CAD build for the part. Positions are in the model's coordinates, mm. Face numbers are marked on the shaded views. A direction names the side the tool comes from. Coordinates: 2 decimals unless noted, no trailing zeros. Loops run counter-clockwise (first coordinate to the right, second up) from the corner with the lowest first, then second, coordinate; pieces in that order, holes last. Notation, with made-up numbers: (-34, 60) -> (-10, 60) arc R20 ccw to (-10, 77) -> close; hole circle Ø6 at (13.25, -3). An arc over 180 degrees is marked (long way). Write each question's results on one line, items separated by ' | '.
Autodesk Fusion 360 part; units mm, degrees
sketch "Sketch1" plane through (0, 0, 0) normal (0, 1, 0) x (1, 0, 0)
  circle A0 centre (0, 0) radius 1.75
  circle A1 centre (50, 0) radius 1.75
  circle A2 centre (0, -50) radius 1.75
  circle A3 centre (50, -50) radius 1.75
  circle A4 centre (25, -25) radius 4.5
  line L0 (-5, 5) -> (55, 5)
  line L1 (55, 5) -> (55, -55)
  line L2 (55, -55) -> (-5, -55)
  line L3 (-5, -55) -> (-5, 5)
  dimension "d1" = 50
  dimension "d2" = 50
  dimension "d3" = 3.5
  dimension "d4" = 3.5
  dimension "d5" = 3.5
  dimension "d6" = 3.5
  dimension "d7" = 9
extrude "Extrude1" add sketch "Sketch1" along normal blind 4 contours A4 | L0 L1 L2 L3
sketch "Sketch2" plane through (0, 4, 0) normal (0, 1, 0) x (-1, 0, 0)
  circle A0 centre (0, 0) radius 1.75
  circle A1 centre (-50, 0) radius 1.75
  circle A2 centre (0, 50) radius 1.75
  circle A3 centre (-50, 50) radius 1.75
  line L0 (5, 55) -> (-55, 55)
  line L1 (-55, 55) -> (-55, -5)
  line L2 (-55, -5) -> (5, -5)
  line L3 (5, -5) -> (5, 55)
  circle A4 centre (0, 0) radius 3.25
  circle A5 centre (-50, 0) radius 3.25
  circle A6 centre (0, 50) radius 3.25
  circle A7 centre (-50, 50) radius 3.25
  dimension "d10" = 6.5
  dimension "d11" = 6.5
  dimension "d12" = 6.5
  dimension "d13" = 6.5
extrude "Extrude2" add sketch "Sketch2" along normal blind 0.5 contours L0 L1 L2 L3
extrude "Extrude3" cut 1 faces at (-2.7314, 4, -0.2484) along direction (0, -1, 0) blind 2
extrude "Extrude4" cut 1 faces at (-2.7314, 4, 49.7516) along direction (0, -1, 0) blind 2
sketch "Sketch3" plane through (0, 4, 0) normal (0, 1, 0) x (-1, 0, 0)
  circle A0 centre (-50, 0) radius 3.25
  circle A1 centre (-50, 0) radius 1.75
extrude "Extrude5" cut sketch "Sketch3" against normal blind 2
extrude "Extrude6" cut 1 faces at (47.2686, 4, 49.7516) along direction (0, -1, 0) blind 2
sketch "Sketch4" plane through (0, 4.5, 0) normal (0, 1, 0) x (-1, 0, 0)
  circle A0 centre (-50, 50) radius 3.25
  circle A1 centre (-50, 0) radius 3.25
  circle A2 centre (0, 50) radius 3.25
  circle A3 centre (0, 0) radius 3.25
  line L0 (5, -5) -> (5, 55)
  line L1 (5, 55) -> (-55, 55)
  line L2 (-55, 55) -> (-55, -5)
  line L3 (-55, -5) -> (5, -5)
  line L4 (-24, 3) -> (-26, 3)
  line L5 (-10.0926, 8.7898) -> (-11.6247, 7.5042)
  line L6 (-3.1606, 22.1645) -> (-3.5079, 20.1949)
  line L7 (-6.4474, 36.866) -> (-5.4474, 35.134)
  line L8 (-18.4152, 46.0153) -> (-16.5359, 45.3312)
  line L9 (-33.4641, 45.3312) -> (-31.5848, 46.0153)
  line L10 (-44.5526, 35.134) -> (-43.5526, 36.866)
  line L11 (-46.4921, 20.1949) -> (-46.8394, 22.1645)
  line L12 (-38.3753, 7.5042) -> (-39.9074, 8.7898)
  circle A4 centre (-25, 25) radius 15
  line L13 (-11.6247, 7.5042) -> (-16.1457, 12.8921)
  line L14 (-14.6136, 14.1777) -> (-10.0926, 8.7898)
  line L15 (-24, 10.0334) -> (-24, 3)
  line L16 (-26, 3) -> (-26, 10.0334)
  line L17 (-33.8543, 12.8921) -> (-38.3753, 7.5042)
  line L18 (-39.9074, 8.7898) -> (-35.3864, 14.1777)
  line L19 (-39.5656, 21.4163) -> (-46.4921, 20.1949)
  line L20 (-46.8394, 22.1645) -> (-39.9129, 23.3859)
  line L21 (-38.4615, 31.6173) -> (-44.5526, 35.134)
  line L22 (-43.5526, 36.866) -> (-37.4615, 33.3493)
  line L23 (-31.0586, 38.722) -> (-33.4641, 45.3312)
  line L24 (-31.5848, 46.0153) -> (-29.1792, 39.4061)
  line L25 (-20.8208, 39.4061) -> (-18.4152, 46.0153)
  line L26 (-16.5359, 45.3312) -> (-18.9414, 38.722)
  line L27 (-12.5385, 33.3493) -> (-6.4474, 36.866)
  line L28 (-5.4474, 35.134) -> (-11.5385, 31.6173)
  line L29 (-10.0871, 23.3859) -> (-3.1606, 22.1645)
  line L30 (-3.5079, 20.1949) -> (-10.4344, 21.4163)
  line L31 (-25.8167, 5.0167) -> (-26, 3) construction
  arc A5 (-26, 5.025) -> (-25.8167, 5.0167) centre (-25, 25) ccw
  dimension "d27" = 30
extrude "Extrude7" add sketch "Sketch4" along normal blind 9.5 contours L4 A4 L15 L16 | A4 | L5 A4 L13 L14 | L12 A4 L17 L18 | L6 A4 L29 L30 | L11 A4 L19 L20 | L10 A4 L21 L22 | L7 A4 L27 L28 | L9 A4 L23 L24 | L8 A4 L25 L26
extrude "Extrude8" add 1 faces at (24.6667, 7.6667, 3) along direction (0, 0, -1) blind 2.5
chamfer "Chamfer1" distance 9.5 angle 45 1 edges at (25, 14, 0.5)
extrude "Extrude9" add 1 faces at (10.6033, 7.6667, 8.3613) along direction (-0.642788, 0, -0.766044) blind 2.5
extrude "Extrude10" add 1 faces at (3.2763, 7.6667, 21.508) along direction (-0.984808, 0, -0.173648) blind 2.5
extrude "Extrude11" add 1 faces at (6.1141, 7.6667, 36.2887) along direction (-0.866025, 0, 0.5) blind 2.5
extrude "Extrude12" add 1 faces at (17.7888, 7.6667, 45.7872) along direction (-0.34202, 0, 0.939693) blind 2.5
extrude "Extrude13" add 1 faces at (32.8377, 7.6667, 45.5592) along direction (0.34202, 0, 0.939693) blind 2.5
extrude "Extrude14" add 1 faces at (44.2192, 7.6667, 35.7113) along direction (0.866025, 0, 0.5) blind 2.5
extrude "Extrude15" add 1 faces at (46.6079, 7.6667, 20.8515) along direction (0.984808, 0, -0.173648) blind 2.5
extrude "Extrude16" add 1 faces at (38.886, 7.6667, 7.9328) along direction (0.642788, 0, -0.766044) blind 2.5
chamfer "Chamfer2" distance 9.5 angle 45 8 edges at (49.1278, 14, 20.7456) (40.7483, 14, 6.2319) (46.2176, 14, 37.25) (9.2517, 14, 6.2319) (33.3795, 14, 48.0225) (16.6205, 14, 48.0225) (3.7824, 14, 37.25) (0.8722, 14, 20.7456)
sketch "Sketch5" plane through (0, 14, 0) normal (0, 1, 0) x (-1, 0, 0)
  line L0 (-10.4015, 21.4105) -> (-10.0542, 23.3801)
  line L1 (-10.0542, 23.3801) -> (-10.0871, 23.3859)
  arc A0 (-10.0871, 23.3859) -> (-11.5385, 31.6173) centre (-25, 25) ccw
  line L2 (-11.5385, 31.6173) -> (-11.5096, 31.634)
  line L3 (-11.5096, 31.634) -> (-12.5096, 33.366)
  line L4 (-12.5096, 33.366) -> (-12.5385, 33.3493)
  arc A1 (-12.5385, 33.3493) -> (-18.9414, 38.722) centre (-25, 25) ccw
  line L5 (-18.9414, 38.722) -> (-18.93, 38.7534)
  line L6 (-18.93, 38.7534) -> (-20.8094, 39.4374)
  line L7 (-20.8094, 39.4374) -> (-20.8208, 39.4061)
  arc A2 (-20.8208, 39.4061) -> (-29.1792, 39.4061) centre (-25, 25) ccw
  line L8 (-29.1792, 39.4061) -> (-29.1906, 39.4374)
  line L9 (-29.1906, 39.4374) -> (-31.07, 38.7534)
  line L10 (-31.07, 38.7534) -> (-31.0586, 38.722)
  arc A3 (-31.0586, 38.722) -> (-37.4615, 33.3493) centre (-25, 25) ccw
  line L11 (-37.4615, 33.3493) -> (-37.4904, 33.366)
  line L12 (-37.4904, 33.366) -> (-38.4904, 31.634)
  line L13 (-38.4904, 31.634) -> (-38.4615, 31.6173)
  arc A4 (-38.4615, 31.6173) -> (-39.9129, 23.3859) centre (-25, 25) ccw
  line L14 (-39.9129, 23.3859) -> (-39.9458, 23.3801)
  line L15 (-39.9458, 23.3801) -> (-39.5985, 21.4105)
  line L16 (-39.5985, 21.4105) -> (-39.5656, 21.4163)
  arc A5 (-39.5656, 21.4163) -> (-35.3864, 14.1777) centre (-25, 25) ccw
  line L17 (-35.3864, 14.1777) -> (-35.4079, 14.1521)
  line L18 (-35.4079, 14.1521) -> (-33.8758, 12.8665)
  line L19 (-33.8758, 12.8665) -> (-33.8543, 12.8921)
  arc A6 (-33.8543, 12.8921) -> (-26, 10.0334) centre (-25, 25) ccw
  line L20 (-26, 10.0334) -> (-26, 10)
  line L21 (-26, 10) -> (-24, 10)
  line L22 (-24, 10) -> (-24, 10.0334)
  arc A7 (-24, 10.0334) -> (-16.1457, 12.8921) centre (-25, 25) ccw
  line L23 (-16.1457, 12.8921) -> (-16.1242, 12.8665)
  line L24 (-16.1242, 12.8665) -> (-14.5921, 14.1521)
  line L25 (-14.5921, 14.1521) -> (-14.6136, 14.1777)
  arc A8 (-14.6136, 14.1777) -> (-10.4344, 21.4163) centre (-25, 25) ccw
  line L26 (-10.4344, 21.4163) -> (-10.4015, 21.4105)
  circle A9 centre (-25, 25) radius 4.5
  dimension "d50" = 9
extrude "Extrude17" cut sketch "Sketch5" against normal blind 12 contours A9
chamfer "Chamfer3" distance 1 angle 45 1 edges at (29.1955, 14, 26.6273)
sketch "Sketch6" plane through (55, 0, 0) normal (1, 0, 0) x (0, 0, -1)
  line L0 (-55, 0) -> (5, 0)
  line L1 (5, 0) -> (5, 4.5)
  line L2 (5, 4.5) -> (-55, 4.5)
  line L3 (-55, 4.5) -> (-55, 0)
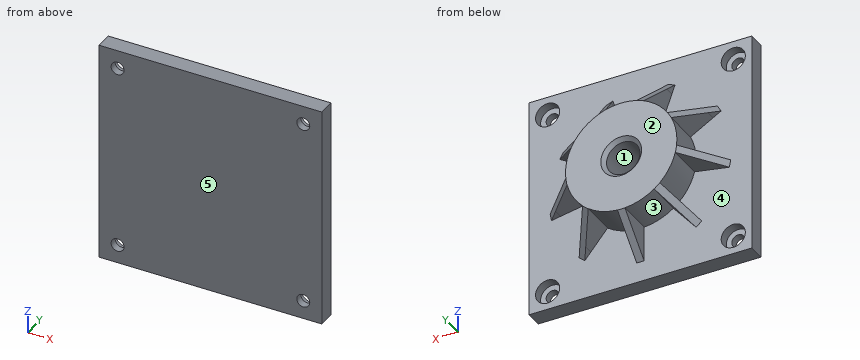
Q1. Cut at B-B on z = 50. Write the cut outline in (x, y), and give its area (4 significant figures).
Results are:
outline: (-5, 0) -> (-1.75, 0) -> (-1.75, 2) -> (-3.25, 2) -> (-3.25, 4.5) -> (-5, 4.5) -> close; (1.75, 0) -> (48.25, 0) -> (48.25, 2) -> (46.75, 2) -> (46.75, 4.5) -> (3.25, 4.5) -> (3.25, 2) -> (1.75, 2) -> close; (51.75, 0) -> (55, 0) -> (55, 4.5) -> (53.25, 4.5) -> (53.25, 2) -> (51.75, 2) -> close | area: 223.5 mm^2
Q2. Cut at A-A on x = 50. Write the cut outline in (y, z).
Results are:
outline: (0, -5) -> (4.5, -5) -> (4.5, -3.25) -> (2, -3.25) -> (2, -1.75) -> (0, -1.75) -> close; (0, 1.75) -> (2, 1.75) -> (2, 3.25) -> (4.5, 3.25) -> (4.5, 46.75) -> (2, 46.75) -> (2, 48.25) -> (0, 48.25) -> close; (0, 51.75) -> (2, 51.75) -> (2, 53.25) -> (4.5, 53.25) -> (4.5, 55) -> (0, 55) -> close
Q3. Drop flat-ended pins along their axis: pin 1 (4.5 mm diameter, centred on x = 50, z = 50, fed in from +Y); pin 2 (4 mm diameter, centred on x = 28.5, z = 17, fed in from -Y); pin 3 (4 mm diameter, centred on x = 7, z = 26.5, fed in from +Y); pin 4 (2 mm diameter, centred on y = 9.5, z = 5.5, fed in from +X). Give the stop position or say it passes through.
Results are:
pin 1: y = 2 | pin 2: y = 0 | pin 3: y = 4.5 | pin 4: x = 26
Q4. Cut at C-C on z = 25. Write the cut outline in (x, y).
Results are:
outline: (-5, 0) -> (55, 0) -> (55, 4.5) -> (40, 4.5) -> (40, 14) -> (30.5, 14) -> (29.5, 13) -> (29.5, 2) -> (20.5, 2) -> (20.5, 13) -> (19.5, 14) -> (10, 14) -> (10, 4.5) -> (-5, 4.5) -> close
Q5. Pull direction X, two halves, no side cores. Call the marked faces 1 and 2: +X half, -X half, draft (parallel to the pull), parting line (faces both ways), or undercut.
Results are:
face 1: undercut | face 2: draft
Q6. Wall check: L1, parallel to Z at x = 50, y = 2.65; L2, parallel to Z at x = 50, y = 0.55; L3, parallel to X at y = 4.25, z = 1.5. Give the ranges that are in metal, low to high. Write a range as from..to.
Results are:
L1: -5..-3.25, 3.25..46.75, 53.25..55 | L2: -5..-1.75, 1.75..48.25, 51.75..55 | L3: -5..-2.88, 2.88..47.12, 52.88..55
Q7. Which spindle directions (+Z, -Z, +X, -X, +Y, -Y) get a long thin tool onto all of the face, cutting with end or side? Do the marked faces 3, 4 and 5. Say none if no direction does.
Results are:
face 3: -Z, +Y | face 4: +Y | face 5: +Z, -Z, +X, -X, -Y
